from build123d import *
from build123d import SkipClean  # not in build123d's __all__

# Parameters (mm, degrees)
F1_DEPTH  = 1.6
F2_W      = 25
F2_H      = 16
F3_DEPTH  = 1.6
F5_DEPTH  = 25
F6_R      = 5
F8_R      = 5.5
F9_DEPTH  = 25
F12_R     = 8.5
F12_R_2   = 5.5
F13_DEPTH = 2
F15_DEPTH = 4.2
F17_DEPTH = 1.6
F19_W     = 294.2
F19_H     = 29.2
F19_W_2   = 50.2
F19_H_2   = 13.2
F20_DEPTH = 0.4


# Not quite as in the source:
# - two fillets or chamfers of one size are made in one step
# - after a boolean that leaves OpenCascade's solid faulty, fix() repairs it


with BuildPart() as f1:
    # F0 (on Front) → F1 (new body)
    with BuildSketch(Plane.XZ):
        with BuildLine():
            ThreePointArc((155.5, 65.5), (152.5710678119, 72.5710678119), (145.5, 75.5))
            Line((145.5, 75.5), (-145.5, 75.5))
            ThreePointArc((-145.5, 75.5), (-152.5710678119, 72.5710678119), (-155.5, 65.5))
            Line((-155.5, 65.5), (-155.5, -65.5))
            ThreePointArc((-155.5, -65.5), (-152.5710678119, -72.5710678119), (-145.5, -75.5))
            Line((-145.5, -75.5), (145.5, -75.5))
            ThreePointArc((145.5, -75.5), (152.5710678119, -72.5710678119), (155.5, -65.5))
            Line((155.5, -65.5), (155.5, 65.5))
        make_face()
        with BuildLine():
            Line((-135.5, 60.5), (135.5, 60.5))
            ThreePointArc((135.5, 60.5), (139.0355339059, 59.0355339059), (140.5, 55.5))
            Line((140.5, 55.5), (140.5, -30.5))
            ThreePointArc((140.5, -30.5), (137.5710678119, -37.5710678119), (130.5, -40.5))
            Line((130.5, -40.5), (-135.5, -40.5))
            ThreePointArc((-135.5, -40.5), (-139.0355339059, -39.0355339059), (-140.5, -35.5))
            Line((-140.5, -35.5), (-140.5, 55.5))
            ThreePointArc((-140.5, 55.5), (-139.0355339059, 59.0355339059), (-135.5, 60.5))
        make_face(mode=Mode.SUBTRACT)
    extrude(amount=F1_DEPTH)

    # F2 (on face) → F3 (join, through all)
    with BuildSketch(Plane.XZ.offset(1.6)):
        with Locations((-88.5, 52.5)):
            Rectangle(F2_W, F2_H)
        with Locations((88.5, 52.5)):
            Rectangle(F2_W, F2_H)
    extrude(amount=-F3_DEPTH)

    # F4 (on face) → F5 (cut)
    with BuildSketch(Plane.XZ.offset(1.6)):
        Polygon((101, 64.5), (101, 60.5), (101, 55.5), (140.5, 55.5), (140.5, 64.5), align=None)
    extrude(amount=-F5_DEPTH, mode=Mode.SUBTRACT)

    # F6
    f6_edges = [f1.edges().sort_by_distance(p)[0] for p in [
        (-101, -0.8, 44.5),
        (-101, -0.8, 60.5),
        (-76, -0.8, 44.5),
        (-76, -0.8, 60.5),
        (101, -0.8, 44.5),
        (76, -0.8, 44.5),
        (76, -0.8, 60.5),
        (140.5, -0.8, 64.5),
        (101, -0.8, 64.5),
    ]]
    fillet(f6_edges, radius=F6_R)

    # F8 (on face) → F9 (cut)
    with BuildSketch(Plane.XZ.offset(1.6)):
        with Locations((-88.5, 56.5)):
            Circle(F8_R)
        with Locations((88.5, 56.5)):
            Circle(F8_R)
    extrude(amount=-F9_DEPTH, mode=Mode.SUBTRACT)

    # F12 (on face) → F13 (join)
    with BuildSketch(Plane(origin=(0, 0, 0), x_dir=(-1, 0, 0), z_dir=(0, 1, 0))):
        with Locations((-88.5, 56.5)):
            Circle(F12_R)
        with Locations((-88.5, 56.5)):
            Circle(F12_R_2, mode=Mode.SUBTRACT)
        with Locations((88.5, 56.5)):
            Circle(F12_R)
        with Locations((88.5, 56.5)):
            Circle(F12_R_2, mode=Mode.SUBTRACT)
    with SkipClean():  # cleaning this boolean's faces spoils the solid; the shape is the same uncleaned
        extrude(amount=F13_DEPTH)

    # F14 (on face) → F15 (join)
    with BuildSketch(Plane(origin=(0, 0, 0), x_dir=(-1, 0, 0), z_dir=(0, 1, 0))):
        with BuildLine():
            ThreePointArc((-145.5, 75.5), (-152.5710678119, 72.5710678119), (-155.5, 65.5))
            Line((-155.5, 65.5), (-155.5, -65.5))
            Line((-155.5, -65.5), (-153.5, -65.5))
            Line((-153.5, -65.5), (-153.5, 65.5))
            ThreePointArc((-153.5, 65.5), (-151.1568542495, 71.1568542495), (-145.5, 73.5))
            Line((-145.5, 73.5), (145.5, 73.5))
            ThreePointArc((145.5, 73.5), (151.1568542495, 71.1568542495), (153.5, 65.5))
            Line((153.5, 65.5), (153.5, -65.5))
            Line((153.5, -65.5), (155.5, -65.5))
            Line((155.5, -65.5), (155.5, 65.5))
            ThreePointArc((155.5, 65.5), (152.5710678119, 72.5710678119), (145.5, 75.5))
            Line((145.5, 75.5), (-145.5, 75.5))
        make_face()
    extrude(amount=F15_DEPTH)

    add(f1.part.fix(), mode=Mode.REPLACE)

    # F16 (on face) → F17 (join)
    with BuildSketch(Plane(origin=(0, 4.2, 0), x_dir=(-1, 0, 0), z_dir=(0, 1, 0))):
        Polygon((-153.5, 31), (-153.5, -31), (-146.5, -31), (-146.5, 22.6577248518), align=None)
        Polygon((146.5, -31), (153.5, -31), (153.5, 31), (146.5, 22.6577248518), align=None)
    extrude(amount=-F17_DEPTH)

    # F19 (on face) → F20 (cut)
    with BuildSketch(Plane.XZ.offset(1.6)):
        with Locations((0, -58.5)):
            Rectangle(F19_W, F19_H)
        with Locations((0, 68)):
            Rectangle(F19_W_2, F19_H_2)
    extrude(amount=-F20_DEPTH, mode=Mode.SUBTRACT)


solid = f1.part
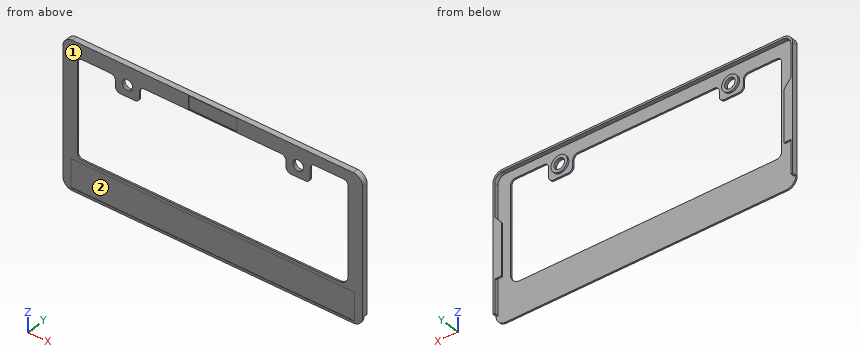
Geometry check sheet. Reference: the model listing, model coordinates, mm. Face numbers are marked on the shaded views. Give positions to 0.01 mm unless a question says otherwise; leave off trailing zeros. Order: outer loops, then holes, each group sorted by start corner. A loop starts at its lowest first (then second) coordinate and runs counter-clockwise, first axis right, second up. Notation, with made-up numbers: (63, 7.25) - (68, 7.25) arc R17 cw to (68, 13.25) - close; hole circle Ø1 at (-9, 55.25). An arc over 180 degrees is marked (long way). Answer as a JSON object with one key per item and string values.
(1) Cross-section at B-B (z = -3). Record the cut outline in (x, y), then the cut area to 3 significant figures.
Report:
{"outline": "(-155.5, -1.6) - (-140.5, -1.6) - (-140.5, 0) - (-153.5, 0) - (-153.5, 2.6) - (-146.5, 2.6) - (-146.5, 4.2) - (-155.5, 4.2) - close; (140.5, -1.6) - (155.5, -1.6) - (155.5, 4.2) - (146.5, 4.2) - (146.5, 2.6) - (153.5, 2.6) - (153.5, 0) - (140.5, 0) - close", "area": "87.2 mm^2"}
(2) Cross-section at C-C (x = -46). Record the cut outline in (y, z).
Report:
{"outline": "(-1.6, -75.5) - (0, -75.5) - (0, -40.5) - (-1.6, -40.5) - (-1.6, -43.9) - (-1.2, -43.9) - (-1.2, -73.1) - (-1.6, -73.1) - close; (-1.6, 60.5) - (0, 60.5) - (0, 73.5) - (4.2, 73.5) - (4.2, 75.5) - (-1.6, 75.5) - close"}
(3) Cross-section at A-A (x = -88.5). Record the cut outline in (y, z).
Report:
{"outline": "(-1.6, -75.5) - (0, -75.5) - (0, -40.5) - (-1.6, -40.5) - (-1.6, -43.9) - (-1.2, -43.9) - (-1.2, -73.1) - (-1.6, -73.1) - close; (-1.6, 44.5) - (0, 44.5) - (0, 48) - (2, 48) - (2, 51) - (-1.6, 51) - close; (-1.6, 62) - (2, 62) - (2, 65) - (0, 65) - (0, 73.5) - (4.2, 73.5) - (4.2, 75.5) - (-1.6, 75.5) - close"}
(4) Draft check along X on the marked faces 1 and 2. Enter one of: released by +X, released by -X, zero draft, split by the parting line, or undercut.
Report:
{"face 1": "zero draft", "face 2": "undercut"}
(5) Material ranges on line 1 (Z direction, x = -88.5, y = 0.45); line 2 (X direction, y = 2.8, z = 10); line 3 (X direction, y = 1.9, z = 4.5), recorded low to high.
Report:
{"line 1": "48 to 51, 62 to 65, 73.5 to 75.5", "line 2": "-155.5 to -146.5, 146.5 to 155.5", "line 3": "-155.5 to -153.5, 153.5 to 155.5"}
(6) Cross-section at D-D (x = 116). Record the cut outline in (y, z).
Report:
{"outline": "(-1.6, -75.5) - (0, -75.5) - (0, -40.5) - (-1.6, -40.5) - (-1.6, -43.9) - (-1.2, -43.9) - (-1.2, -73.1) - (-1.6, -73.1) - close; (-1.6, 64.5) - (0, 64.5) - (0, 73.5) - (4.2, 73.5) - (4.2, 75.5) - (-1.6, 75.5) - close"}
(7) Depth check by flat-ended pin: pin 1 Ø9 at (x, z) = (88.5, 56.5) entering from -Y; pin 2 Ø0.6 at (x, y) = (154.5, 3) entering from -Z; pin 3 Ø0.5 at (x, y) = (-151.5, 3) entering from -Z; pin 4 Ø9 at (x, z) = (-23.5, -52) entering from -Y. Enter the tip coordinate at first touch or a pass-through.
Report:
{"pin 1": "through", "pin 2": "z = -65.5", "pin 3": "z = -31", "pin 4": "y = -1.2"}
